For this review, take the finished solid that the model builds, in its own axes (mm). Face numbers are marked on the shaded views. A direction names the side the tool comes from. Give positions to 0.01 mm unless a question says otherwise; leave off trailing zeros. Order: outer loops, then holes, each group sorted by start corner. A loop starts at its lowest first (then second) coordinate and runs counter-clockwise, first axis right, second up. Notation, with made-up numbers: (-18.5, -12) - (20.5, -12) arc R25 cw to (20.5, 15) - close; hole circle Ø1 at (15, 56). An arc over 180 degrees is marked (long way). Put each result on its own line as item: value. Start each with the question number.
```python
from build123d import *

# Parameters (mm, degrees)
SKETCH_1_W          = 215
SKETCH_1_H          = 115
EXTRUDE_1_DEPTH     = 51
CUT_EXTRUDE_1_DEPTH = 20


with BuildPart() as part:
    # Эскиз1 → Бобышка-Вытянуть1 (new body)
    with BuildSketch(Plane(origin=(0, 0, 0), x_dir=(1, 0, 0), z_dir=(0, 1, 0))):
        Rectangle(SKETCH_1_W, SKETCH_1_H)
    extrude(amount=EXTRUDE_1_DEPTH)

    # Эскиз3 → Вырез-Вытянуть1 (cut)
    with BuildSketch(Plane(origin=(107.5, 0, 0), x_dir=(0, 0, -1), z_dir=(1, 0, 0))):
        Polygon((-56, 51), (56, 51), (56, 24), (56, 8), (38, 8), (38, 24), (-38, 24), (-38, 8), (-56, 8), (-56, 24), align=None)
    extrude(amount=-CUT_EXTRUDE_1_DEPTH, mode=Mode.SUBTRACT)


solid = part.part
```
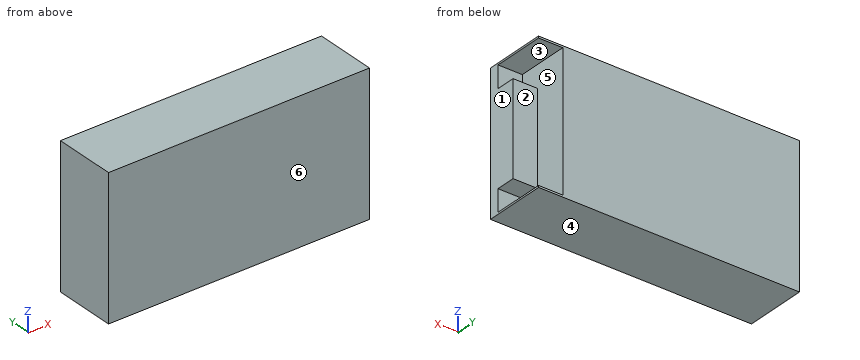
1. Add section B-B, the plane z = 47.5. Give the boundary of the cut face in (x, y).
2. Clearance check with flat-ended pins moving along their axes: pin 1 (5.5 mm diameter, centred on x = 94, z = 47.5, fed in from +Y); pin 2 (16 mm diameter, centred on x = 101, z = -10.5, fed in from +Y). State where each tip first meets the part, or that it passes through.
3. Wall thickness on line 1 (X direction, y = 32, z = 51); line 2 (Y direction, x = 92, z = 2): over which ranges is each line inside the solid? List them lowest first. Write a range as from..to.
4. Add section D-D, the plane z = -6.5. Give the boundary of the cut face in (x, y).
5. Add section C-C, the plane y = 13. Give the boundary of the cut face in (x, z).
6. Tool access review of the marked faces 1 and 2: name each direction out of +Z, -Z, +X, -X, +Y, -Y from which nothing blocks a thin tool from reaching the whole face with its end or side.
7. The part is to be moulded in two halves that separate along Z. For the marked faces 3, 4, 5 and 6, say which applies: released by +Z, released by -Z, zero draft, split by the parting line, or undercut.
8. Add section A-A, the plane y = 39.5. Give the boundary of the cut face in (x, z), then the cut area to 3 significant figures.
Found:
1. outline: (-107.5, 0) - (107.5, 0) - (107.5, 8) - (87.5, 8) - (87.5, 51) - (-107.5, 51) - close
2. pin 1: stops at y = 8
2. pin 2: stops at y = 24
3. line 1: x = -107.5..87.5
3. line 2: y = 0..24
4. outline: (-107.5, 0) - (107.5, 0) - (107.5, 24) - (87.5, 24) - (87.5, 51) - (-107.5, 51) - close
5. outline: (-107.5, -57.5) - (107.5, -57.5) - (107.5, -56) - (87.5, -56) - (87.5, -38) - (107.5, -38) - (107.5, 38) - (87.5, 38) - (87.5, 56) - (107.5, 56) - (107.5, 57.5) - (-107.5, 57.5) - close
6. face 1: +Z, -Z, +X, +Y, -Y
6. face 2: +X, +Y
7. face 3: undercut
7. face 4: released by -Z
7. face 5: undercut
7. face 6: zero draft
8. outline: (-107.5, -57.5) - (107.5, -57.5) - (107.5, -56) - (87.5, -56) - (87.5, 56) - (107.5, 56) - (107.5, 57.5) - (-107.5, 57.5) - close
8. area: 22,500 mm^2
